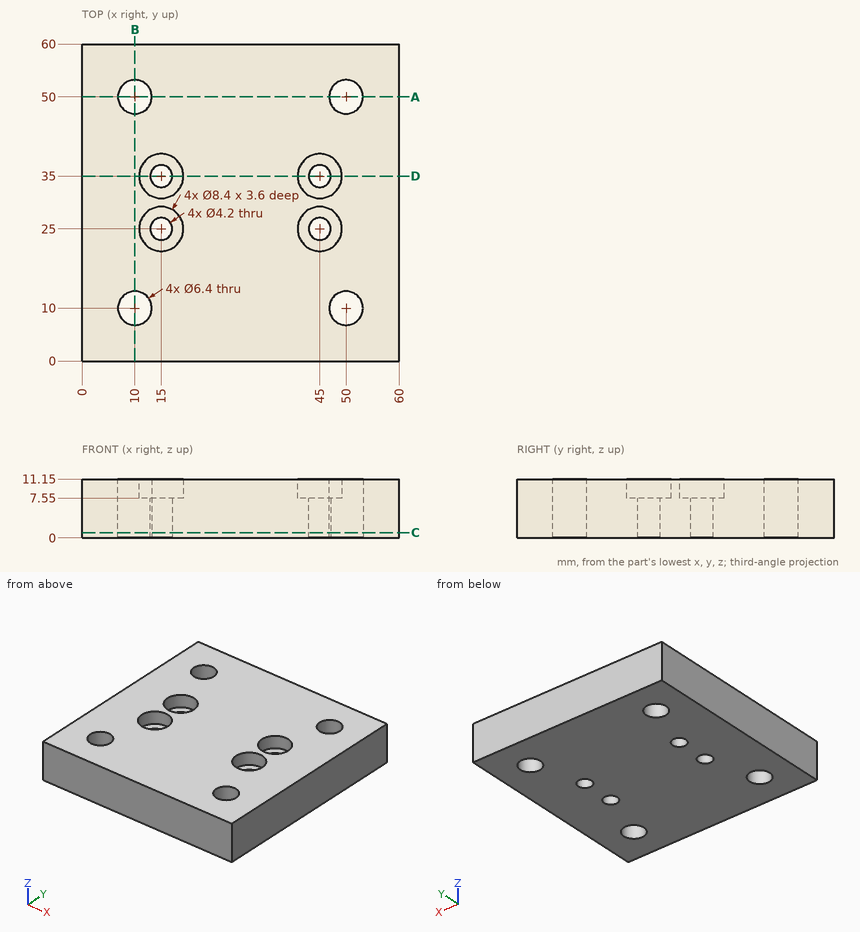
Verification items for this drawing (mm, ordinates from the low corner). Give positions to 0.01 mm unless a question says otherwise; leave off trailing zeros. Loops run counter-clockwise (first coordinate to the right, second up) from the corner with the lowest first, then second, coordinate; pieces in that order, holes last. Notation, with made-up numbers: M 39.25,52.5 L 46.25,52.5 A17 cw 46.25,73.5 Z; hole C -4.75,50.5 d8. An arc over 180 degrees is marked long. Write item = value, one per line.
(1) Sectioned sample at A-A, the plane y = 50. Record the cut outline in (x, z), plus the area to 3 significant figures.
Answer below:
outline = M 0,0 L 6.8,0 L 6.8,11.15 L 0,11.15 Z; M 13.2,0 L 46.8,0 L 46.8,11.15 L 13.2,11.15 Z; M 53.2,0 L 60,0 L 60,11.15 L 53.2,11.15 Z
area = 526 mm2
(2) Material ranges on line 1 (Y direction, x = 10, z = 5); line 2 (Y direction, x = 8.5, z = 1.25); line 3 (X direction, y = 7.5, z = 0.75), recorded low to high. Write a range as [from, to].
Answer below:
line_1 = [0, 6.8], [13.2, 46.8], [53.2, 60]
line_2 = [0, 7.17], [12.83, 47.17], [52.83, 60]
line_3 = [0, 8], [12, 48], [52, 60]
(3) Sectioned sample at D-D, the plane y = 35. Record the cut outline in (x, z), plus the area to 3 significant figures.
Answer below:
outline = M 0,0 L 12.9,0 L 12.9,7.55 L 10.8,7.55 L 10.8,11.15 L 0,11.15 Z; M 17.1,0 L 42.9,0 L 42.9,7.55 L 40.8,7.55 L 40.8,11.15 L 19.2,11.15 L 19.2,7.55 L 17.1,7.55 Z; M 47.1,0 L 60,0 L 60,11.15 L 49.2,11.15 L 49.2,7.55 L 47.1,7.55 Z
area = 545 mm2
(4) Gauge pin test, flat ends, axial feed: pin 1 Ø3.5 at (x, y) = (45, 35) entering from +Z; pin 2 Ø6.5 at (x, y) = (15, 35) entering from +Z. Record the tip position at first contact, or that the pin passes through.
Answer below:
pin_1 = through
pin_2 = 7.55
(5) Sectioned sample at C-C, the plane z = 1. State how many separate pieces and enclosed holes the cut face has, plus the area to 3 significant figures.
Answer below:
separate_pieces = 1
enclosed_holes = 8
area = 3,420 mm2
